```python
from build123d import *

# Parameters (mm, degrees)
SKETCH001_W     = 32.14
SKETCH001_H     = 11.86
PAD_DEPTH       = 27.59
SKETCH002_W     = 4.75
SKETCH002_H     = 11.86
POCKET_DEPTH    = 8.44
SKETCH_W        = 4.75
SKETCH_H        = 11.86
POCKET001_DEPTH = 16.61
SKETCH003_W     = 8.06
SKETCH003_H     = 11.86
POCKET002_DEPTH = 4.36
SKETCH004_R     = 1.295
POCKET003_DEPTH = 2.54
SKETCH005_R     = 1.295
POCKET004_DEPTH = 2.54
SKETCH007_W     = 1.066805
SKETCH007_H     = 1.19
POCKET005_DEPTH = 2.54
SKETCH008_W     = 1.5
SKETCH008_H     = 1.19
POCKET006_DEPTH = 2.54
SKETCH011_W     = 14.58
SKETCH011_H     = 11.86
POCKET007_DEPTH = 4.36
SKETCH012_R     = 5.93
PAD001_DEPTH    = 4.36
SKETCH013_R     = 2.66
PAD002_DEPTH    = 4.36
SKETCH014_R     = 2.38
PAD003_DEPTH    = 1.07
SKETCH015_R     = 3.39
PAD004_DEPTH    = 3.7
PAD005_DEPTH    = 1.48
SKETCH017_R     = 2.29
POCKET008_DEPTH = 1.66
SKETCH018_R     = 1.1
POCKET009_DEPTH = 1.66
SKETCH019_R     = 0.575
PAD006_DEPTH    = 10


with BuildPart() as part:
    # Sketch001 → Pad (new body)
    with BuildSketch(Plane.XZ):
        with Locations((16.07, 5.93)):
            Rectangle(SKETCH001_W, SKETCH001_H)
    extrude(amount=PAD_DEPTH)

    # Sketch002 (on Face6 of Pad) → Pocket (cut)
    with BuildSketch(Plane.XZ.offset(27.59)):
        with Locations((2.375, 5.93)):
            Rectangle(SKETCH002_W, SKETCH002_H)
        with Locations((29.765, 5.93)):
            Rectangle(SKETCH002_W, SKETCH002_H)
    extrude(amount=-POCKET_DEPTH, mode=Mode.SUBTRACT)

    # Sketch (on Face2 of Pocket) → Pocket001 (cut)
    with BuildSketch(Plane(origin=(0, 0, 0), x_dir=(1, 0, 0), z_dir=(0, 1, 0))):
        with Locations((2.375, -5.93)):
            Rectangle(SKETCH_W, SKETCH_H)
        with Locations((29.765, -5.93)):
            Rectangle(SKETCH_W, SKETCH_H)
    extrude(amount=-POCKET001_DEPTH, mode=Mode.SUBTRACT)

    # Sketch003 (on Face8 of Pocket001) → Pocket002 (cut)
    with BuildSketch(Plane.XZ.offset(27.59)):
        with Locations((23.36, 5.93)):
            Rectangle(SKETCH003_W, SKETCH003_H)
    extrude(amount=-POCKET002_DEPTH, mode=Mode.SUBTRACT)

    # Sketch004 (on Face6 of Pocket002) → Pocket003 (cut)
    with BuildSketch(Plane.XZ.offset(19.15)):
        with Locations((29.925, 5.93)):
            Circle(SKETCH004_R)
    extrude(amount=-POCKET003_DEPTH, mode=Mode.SUBTRACT)

    # Sketch005 (on Face12 of Pocket003) → Pocket004 (cut)
    with BuildSketch(Plane.XZ.offset(19.15)):
        with Locations((2.215, 5.93)):
            Circle(SKETCH005_R)
    extrude(amount=-POCKET004_DEPTH, mode=Mode.SUBTRACT)

    # Sketch007 (on Face6 of Pocket004) → Pocket005 (cut)
    with BuildSketch(Plane.XZ.offset(19.15)):
        with Locations((31.6065975, 5.93)):
            Rectangle(SKETCH007_W, SKETCH007_H)
    extrude(amount=-POCKET005_DEPTH, mode=Mode.SUBTRACT)

    # Sketch008 (on Face12 of Pocket005) → Pocket006 (cut)
    with BuildSketch(Plane.XZ.offset(19.15)):
        with Locations((0.75, 5.93)):
            Rectangle(SKETCH008_W, SKETCH008_H)
    extrude(amount=-POCKET006_DEPTH, mode=Mode.SUBTRACT)

    # Sketch011 (on Face10 of Pocket006) → Pocket007 (cut)
    with BuildSketch(Plane.XZ.offset(27.59)):
        with Locations((12.04, 5.93)):
            Rectangle(SKETCH011_W, SKETCH011_H)
    extrude(amount=-POCKET007_DEPTH, mode=Mode.SUBTRACT)

    # Sketch012 (on Face9 of Pocket007) → Pad001 (join)
    with BuildSketch(Plane.XZ.offset(23.23)):
        with Locations((10.73, 5.98)):
            Circle(SKETCH012_R)
    extrude(amount=PAD001_DEPTH)

    # Sketch013 (on Face9 of Pad001) → Pad002 (join)
    with BuildSketch(Plane.XZ.offset(23.23)):
        with Locations((16.67, 5.93)):
            Circle(SKETCH013_R)
    extrude(amount=PAD002_DEPTH)

    # Sketch014 (on Face24 of Pad002) → Pad003 (join)
    with BuildSketch(Plane.XZ.offset(27.59)):
        with Locations((10.68, 5.93)):
            Circle(SKETCH014_R)
    extrude(amount=PAD003_DEPTH)

    # Sketch015 (on Face28 of Pad003) → Pad004 (join)
    with BuildSketch(Plane.XZ.offset(28.66)):
        with Locations((10.68, 5.93)):
            Circle(SKETCH015_R)
    extrude(amount=PAD004_DEPTH)

    # Sketch016 (on Face3 of Pad004) → Pad005 (join)
    with BuildSketch(Plane.XZ.offset(32.36)):
        with BuildLine():
            Line((8.62, 8.58), (8.62, 3.26))
            Line((-3.5526338926, 4.0654001014), (8.62, 3.26))
            ThreePointArc((-3.6067901761, 7.3671849678), (-5.0997771882, 5.691360238), (-3.5526338926, 4.0654001014))
            Line((8.62, 8.58), (-3.6067901761, 7.3671849678))
        make_face()
    extrude(amount=-PAD005_DEPTH)

    # Sketch017 (on Face34 of Pad005) → Pocket008 (cut)
    with BuildSketch(Plane.XZ.offset(32.36)):
        with Locations((10.668875, 5.93)):
            Circle(SKETCH017_R)
    extrude(amount=-POCKET008_DEPTH, mode=Mode.SUBTRACT)

    # Sketch018 (on Face11 of Pocket008) → Pocket009 (cut)
    with BuildSketch(Plane.XZ.offset(30.7)):
        with Locations((10.68, 5.93)):
            Circle(SKETCH018_R)
    extrude(amount=-POCKET009_DEPTH, mode=Mode.SUBTRACT)

    # Sketch019 (on Face23 of Pocket009) → Pad006 (join)
    with BuildSketch(Plane(origin=(4.75, 0, 0), x_dir=(0, 0, -1), z_dir=(-1, 0, 0))):
        with Locations((-5.93, 4.256319)):
            Circle(SKETCH019_R)
        with Locations((-7.12, 4.256319)):
            Circle(SKETCH019_R)
        with Locations((-4.745135, 4.256319)):
            Circle(SKETCH019_R)
    extrude(amount=PAD006_DEPTH)


solid = part.part
```
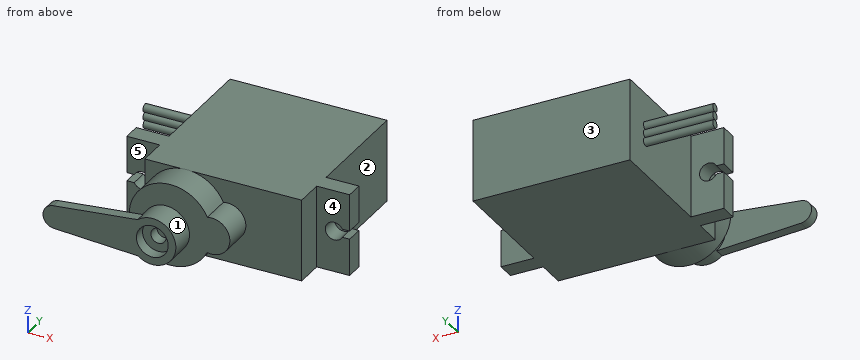
Source: CAD feature listing. Evaluate the final solid. Frame: model axes, mm. Face numbers are marked on the shaded views. A direction names the side the tool comes from. Give positions to 0.01 mm unless a question says otherwise; leave off trailing zeros. Loops run counter-clockwise (first coordinate to the right, second up) from the corner with the lowest first, then second, coordinate; pieces in that order, holes last. Notation, with made-up numbers: (-32, 80.25) -> (26, 80.25) arc R29 cw to (26, 119.25) -> close; hole circle Ø7 at (44, 13.5). An arc over 180 degrees is marked (long way). Use a Markdown table: item, result. Add a question column.
(1) Section query A-A (x = 5.5). Output: boundary loops of the cut face in (y, z) (3 decimals), then the cut area to 3 significant figures.
(2) Section query C-C (x = 17). Output: boundary loops of the cut face in (y, z), then the cut area to 3 significant figures.
(3) Section query D-D (x = 10.73). Output: boundary loops of the cut face in (y, z).
(4) Access query for the marked faces 1, 2, 3, 4 and 5. Directions: +Z, -Z, +X, -X, +Y, -Y. A direction counts if a zero-diameter tool reaches every point of the face in a straight line with its end or side. Return the directions, or none.
(5) Ray query, line 1 (Y direction, x = 13, z = 3.75); line 2 (Z direction, x = 10.68, y = -29.95); line 3 (Y direction, x = 18.5, z = 11.25). Return the intervals inside material, ascending.
(6) Section query B-B (y = -21). Output: boundary loops of the cut face in (x, z), then the cut area to 3 significant figures.
(7) First-contact query: pin 1 Ø1.3 at (y, z) = (-17.5, 8) entering from -X; pin 2 Ø3 at (x, z) = (8.5, 5.5) entering from -Y; pin 3 Ø2.5 at (x, z) = (10.5, 5.5) entering from -Y; pin 4 Ø5 at (x, z) = (31, 6.5) entering from -Y. Flat tips, straight axial feed; report the tip coordinate or a pass-through.
Checked values:
| question | item | result |
|---|---|---|
| 1 | outline | (-32.36, 3.466) -> (-30.88, 3.466) -> (-30.88, 8.271) -> (-32.36, 8.271) -> close; (-27.59, 3.185) -> (-23.23, 3.185) -> (-23.23, 0) -> (0, 0) -> (0, 11.86) -> (-23.23, 11.86) -> (-23.23, 8.775) -> (-27.59, 8.775) -> close |
| 1 | area | 307 mm^2 |
| 2 | outline | (-27.59, 3.29) -> (-23.23, 3.29) -> (-23.23, 0) -> (0, 0) -> (0, 11.86) -> (-23.23, 11.86) -> (-23.23, 8.57) -> (-27.59, 8.57) -> close |
| 2 | area | 299 mm^2 |
| 3 | outline | (-32.36, 2.54) -> (-28.66, 2.54) -> (-28.66, 3.55) -> (-27.59, 3.55) -> (-27.59, 0.05) -> (-23.23, 0.05) -> (-23.23, 0) -> (0, 0) -> (0, 11.86) -> (-23.23, 11.86) -> (-23.23, 11.91) -> (-27.59, 11.91) -> (-27.59, 8.31) -> (-28.66, 8.31) -> (-28.66, 9.32) -> (-32.36, 9.32) -> (-32.36, 8.22) -> (-30.7, 8.22) -> (-30.7, 7.03) -> (-29.04, 7.03) -> (-29.04, 4.83) -> (-30.7, 4.83) -> (-30.7, 3.64) -> (-32.36, 3.64) -> close |
| 4 | face 1 | none |
| 4 | face 2 | +Z, -Z, +X, +Y |
| 4 | face 3 | +Z, -Z, +X, -X, +Y |
| 4 | face 4 | +Z, -Z, +X, -Y |
| 4 | face 5 | +Z, -Z, -X |
| 5 | line 1 | -32.36 to -28.66, -27.59 to 0 |
| 5 | line 2 | 2.54 to 4.83, 7.03 to 9.32 |
| 5 | line 3 | -23.23 to 0 |
| 6 | outline | (4.75, 0) -> (27.39, 0) -> (27.39, 11.86) -> (4.75, 11.86) -> close |
| 6 | area | 269 mm^2 |
| 7 | pin 1 | x = 0 |
| 7 | pin 2 | y = -32.36 |
| 7 | pin 3 | y = -30.7 |
| 7 | pin 4 | y = -19.15 |
